```python
from build123d import *

# Parameters (mm, degrees)
F3_DEPTH = 18.1


with BuildPart() as f1:
    # F0 (on Front) → F1 (revolve)
    with BuildSketch(Plane.XZ):
        with BuildLine():
            Line((0, 21.7), (0, 10.9))
            Line((0, 10.9), (18.1, 10.9))
            Line((18.1, 10.9), (18.1, 21.7))
            ThreePointArc((18.1, 21.7), (9.05, 22.75), (0, 21.7))
        make_face()
    revolve(axis=Axis((10.226779, 0, 0), (1, 0, 0)))

    # F2 (on face) → F3 (cut, through all)
    with BuildSketch(Plane.YZ.offset(18.1)):
        Polygon((1.654276, 10.773735), (0.822951, 12.5), (-0.822951, 12.5), (-1.654276, 10.773735), align=None)
        Polygon((-3.184097, 10.424564), (-4.682093, 11.619176), (-6.165, 10.905046), (-6.165, 8.989036), align=None)
        Polygon((-7.391821, 8.010679), (-9.259792, 8.437032), (-10.285995, 7.150213), (-9.45467, 5.423949), align=None)
        Polygon((-10.135504, 4.010182), (-12.003475, 3.58383), (-12.369723, 1.979194), (-10.871726, 0.784581), align=None)
        Polygon((-10.871726, -0.784581), (-12.369723, -1.979194), (-12.003475, -3.58383), (-10.135504, -4.010182), align=None)
        Polygon((-9.45467, -5.423949), (-10.285995, -7.150213), (-9.259792, -8.437032), (-7.391821, -8.010679), align=None)
        Polygon((-6.165, -8.989036), (-6.165, -10.905046), (-4.682093, -11.619176), (-3.184097, -10.424564), align=None)
        Polygon((-1.654276, -10.773735), (-0.822951, -12.5), (0.822951, -12.5), (1.654276, -10.773735), align=None)
        Polygon((3.184097, -10.424564), (4.682093, -11.619176), (6.165, -10.905046), (6.165, -8.989036), align=None)
        Polygon((7.391821, -8.010679), (9.259792, -8.437032), (10.285995, -7.150213), (9.45467, -5.423949), align=None)
        Polygon((10.135504, -4.010182), (12.003475, -3.58383), (12.369723, -1.979194), (10.871726, -0.784581), align=None)
        Polygon((10.871726, 0.784581), (12.369723, 1.979194), (12.003475, 3.58383), (10.135504, 4.010182), align=None)
        Polygon((9.45467, 5.423949), (10.285995, 7.150213), (9.259792, 8.437032), (7.391821, 8.010679), align=None)
        Polygon((6.165, 8.989036), (6.165, 10.905046), (4.682093, 11.619176), (3.184097, 10.424564), align=None)
    extrude(amount=-F3_DEPTH, mode=Mode.SUBTRACT)


solid = f1.part
```
Part model, mm, in its own coordinate system. Give positions to 0.01 mm unless a question says otherwise; leave off trailing zeros. Use CSV: the item, a comma, the result in double quotes.
Item 1: Pin check, flat tips, straight feed: P1, Ø5, axis at x = 16, y = 0.5, coming from the -Z side; P2, Ø1.3, axis at x = 12, y = 0, coming from the +Z side; P3, Ø10, axis at x = 13, y = 18, coming from the -Z side. Stop position of each tip, or through.
Taken from the geometry:
P1,"stops at z = -22.5"
P2,"stops at z = 22.68"
P3,"stops at z = -18.47"
Item 2: Pull direction Y, two halves, no side cores. Call faces 1 (the face through (18.1, -10, -5)), 2 (the face through (9.177, -8.339, -8.227)): +Y half, -Y half, draft (parallel to the pull), parting line (faces both ways), or undercut.
Taken from the geometry:
face 1,"draft"
face 2,"undercut"
Item 3: Drill centre lines: probe 1 along Y at (x, z) = (2, -11); probe 2 along Y at (x, z) = (6.5, -1.5); probe 3 along Z at (x, y) = (2.75, -7). Where is each one in solid material? Low to high.
Taken from the geometry:
probe 1,"y = -19.19 to -5.97, -3.91 to -1.55, 1.55 to 3.91, 5.97 to 19.19"
probe 2,"y = -22.62 to -11.77, 11.77 to 22.62"
probe 3,"z = -21.11 to -8.36, 8.36 to 21.11"
